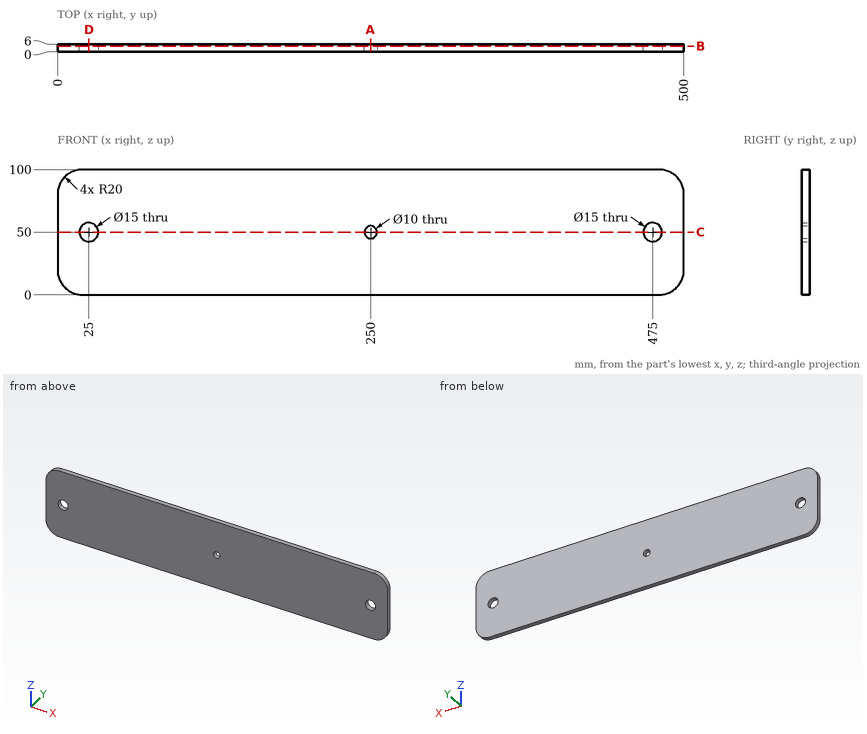
The drawing under review shows one solid part. Ordinate dimensions are in mm from its lowest x, y, z. Round coordinates to 2 decimals unless told otherwise and drop trailing zeros. Write each loop counter-clockwise with the first axis right and the second up, starting at its lowest first coordinate (ties: lowest second). Pieces come first, ordered by that corner, then holes.
(1) Wall thickness on L1, parallel to Z at x = 25, y = 3.05; L2, parallel to Z at x = 250, y = 3.05: over which ranges is each line inside the solid? List them lowest first.
(2) We need section A-A on x = 250. Give the boundary of the cut face in (y, z).
(3) We need section C-C on z = 50. Give the boundary of the cut face in (x, y), and give its area (3 significant figures).
(4) We need section B-B on y = 4.25. Give the boundary of the cut face in (x, z).
(5) We need section D-D on x = 25. Give the boundary of the cut face in (y, z).
Findings below:
1. L1: z = 0 to 42.5, 57.5 to 100
1. L2: z = 0 to 45, 55 to 100
2. outline: (0, 0) - (6, 0) - (6, 45) - (0, 45) - close; (0, 55) - (6, 55) - (6, 100) - (0, 100) - close
3. outline: (0, 0) - (17.5, 0) - (17.5, 6) - (0, 6) - close; (32.5, 0) - (245, 0) - (245, 6) - (32.5, 6) - close; (255, 0) - (467.5, 0) - (467.5, 6) - (255, 6) - close; (482.5, 0) - (500, 0) - (500, 6) - (482.5, 6) - close
3. area: 2,760 mm2
4. outline: (0, 20) arc R20 ccw to (20, 0) - (480, 0) arc R20 ccw to (500, 20) - (500, 80) arc R20 ccw to (480, 100) - (20, 100) arc R20 ccw to (0, 80) - close; hole circle Ø15 at (25, 50); hole circle Ø10 at (250, 50); hole circle Ø15 at (475, 50)
5. outline: (0, 0) - (6, 0) - (6, 42.5) - (0, 42.5) - close; (0, 57.5) - (6, 57.5) - (6, 100) - (0, 100) - close
